Check sheet for the modelled part. Datum: model origin and axes. Units: mm. A direction names the side the tool comes from. Give positions to 0.01 mm unless a question says otherwise; leave off trailing zeros. Order: outer loops, then holes, each group sorted by start corner. A loop starts at its lowest first (then second) coordinate and runs counter-clockwise, first axis right, second up. Notation, with made-up numbers: (53.5, -15.75) -> (59.5, -15.75) arc R8 cw to (59.5, -1.75) -> close; hole circle Ø8 at (10.25, 58.5). An arc over 180 degrees is marked (long way). One line per question, with ' | ' between items.
```python
from build123d import *

# Parameters (mm, degrees)
F0_W     = 25.4
F0_H     = 25.4
F0_W_2   = 15.24
F0_H_2   = 15.24
F1_DEPTH = 5.08
F2_W     = 5.08
F2_H     = 5.08
F3_DEPTH = 15.24
F4_W     = 25.4
F4_H     = 25.4
F4_W_2   = 15.24
F4_H_2   = 15.24
F5_DEPTH = 5.08


with BuildPart() as f1:
    # F0 (on Top) → F1 (new body)
    with BuildSketch(Plane.XY):
        Rectangle(F0_W, F0_H)
        Rectangle(F0_W_2, F0_H_2, mode=Mode.SUBTRACT)
    extrude(amount=F1_DEPTH)

    # F2 (on face) → F3 (join)
    with BuildSketch(Plane.XY.offset(5.08)):
        with Locations((-10.16, 10.16)):
            Rectangle(F2_W, F2_H)
        with Locations((10.16, 10.16)):
            Rectangle(F2_W, F2_H)
        with Locations((10.16, -10.16)):
            Rectangle(F2_W, F2_H)
        with Locations((-10.16, -10.16)):
            Rectangle(F2_W, F2_H)
    extrude(amount=F3_DEPTH)

    # F4 (on face) → F5 (join)
    with BuildSketch(Plane.XY.offset(20.32)):
        Rectangle(F4_W, F4_H)
        Rectangle(F4_W_2, F4_H_2, mode=Mode.SUBTRACT)
    extrude(amount=F5_DEPTH)


solid = f1.part
```
Q1. Section check A-A (z = 5.5). Enter the section's corners in (x, y), and give its area (3 significant figures).
Result sheet:
outline: (-12.7, -12.7) -> (-7.62, -12.7) -> (-7.62, -7.62) -> (-12.7, -7.62) -> close; (-12.7, 7.62) -> (-7.62, 7.62) -> (-7.62, 12.7) -> (-12.7, 12.7) -> close; (7.62, -12.7) -> (12.7, -12.7) -> (12.7, -7.62) -> (7.62, -7.62) -> close; (7.62, 7.62) -> (12.7, 7.62) -> (12.7, 12.7) -> (7.62, 12.7) -> close | area: 103 mm2
Q2. Thickness scan on line 1 (Z direction, x = -11.25, y = 2.5); line 2 (X direction, y = 10.5, z = 12). Record the ranges inside material, lowest first.
Result sheet:
line 1: z = 0 to 5.08, 20.32 to 25.4 | line 2: x = -12.7 to -7.62, 7.62 to 12.7
Q3. Depth check by flat-ended pin: pin 1 Ø6 at (y, z) = (4.5, 20) entering from +X. Enter the tip coordinate at first touch or a pass-through.
Result sheet:
pin 1: stops at x = 12.7
Q4. Mould release check, pull along X, two halves, no side actions. Record for faces 6 (the face through (-10, 0, 20.32)), 7 (the face through (12.7, 8, 13)), 8 (the face through (7.62, -10, 13)), 9 (the face through (0, 7.62, 23)): pulls with the +X half, pulls with the -X half, needs draft (parallel to the pull), parting line crosses it, or undercut.
Result sheet:
face 6: needs draft | face 7: pulls with the +X half | face 8: undercut | face 9: undercut
Q5. Access from +Z, -Z, +X, -X, +Y, -Y to the whole of each face (thin tool, end or side, straight path). Record for faces 1 (the face through (10, -7.62, 13)), 2 (the face through (-12.7, 8, 13)), 3 (the face through (0, -7.62, 3)), 4 (the face through (0, 10, 20.32)), 5 (the face through (8, 12.7, 13)).
Result sheet:
face 1: +X, -X | face 2: +Z, -Z, -X, +Y, -Y | face 3: +Z, -Z | face 4: +Y, -Y | face 5: +Z, -Z, +X, -X, +Y
Q6. Section check C-C (x = 11). Enter the section's corners in (y, z), and give its area (3 significant figures).
Result sheet:
outline: (-12.7, 0) -> (12.7, 0) -> (12.7, 25.4) -> (-12.7, 25.4) -> close; hole (-7.62, 5.08) -> (7.62, 5.08) -> (7.62, 20.32) -> (-7.62, 20.32) -> close | area: 413 mm2
Q7. Section check B-B (y = 3.75). Enter the section's corners in (x, z), and give its area (3 significant figures).
Result sheet:
outline: (-12.7, 0) -> (-7.62, 0) -> (-7.62, 5.08) -> (-12.7, 5.08) -> close; (-12.7, 20.32) -> (-7.62, 20.32) -> (-7.62, 25.4) -> (-12.7, 25.4) -> close; (7.62, 0) -> (12.7, 0) -> (12.7, 5.08) -> (7.62, 5.08) -> close; (7.62, 20.32) -> (12.7, 20.32) -> (12.7, 25.4) -> (7.62, 25.4) -> close | area: 103 mm2
